Could you check a few things on this model? Use its own coordinates, in mm. Round coordinates to 2 decimals unless told otherwise and drop trailing zeros. Loops run counter-clockwise (first coordinate to the right, second up) from the corner with the lowest first, then second, coordinate; pieces in that order, holes last. Notation, with made-up numbers: (84.5, 17) - (138.5, 17) arc R21 ccw to (138.5, 40) - close; hole circle Ø10 at (0.5, 22.25). An arc over 180 degrees is marked (long way). Answer as CSV lines item,"result". Start each with the question number.
1) Suppose I cut it at B-B, the plane x = 45. Write out the boundary of the cut face in (y, z), then the cut area to 3 significant figures.
2) Suppose I cut it at D-D, the plane x = -10. Write out the boundary of the cut face in (y, z).
3) Please list where these lines run through material, in increasing order: line 1 along Z through (x, y) = (-38, 3.1); line 2 along Z through (x, y) = (-29, 1.2); line 3 along X through (y, z) = (1.35, 27).
4) Suppose I cut it at A-A, the plane z = -10. Write out the boundary of the cut face in (x, y).
5) I'm going to push flat-ended pins straight in: pin 1 Ø1 at (x, y) = (42, 3.5) entering from -Z; pin 2 Ø1.4 at (x, y) = (0, 2.5) entering from +Z. Where does each tip first touch, or does it pass through?
6) Suppose I cut it at C-C, the plane y = 2.95. Count the separate pieces of the cut face and the enclosed holes in it, then the cut area to 3 significant figures.
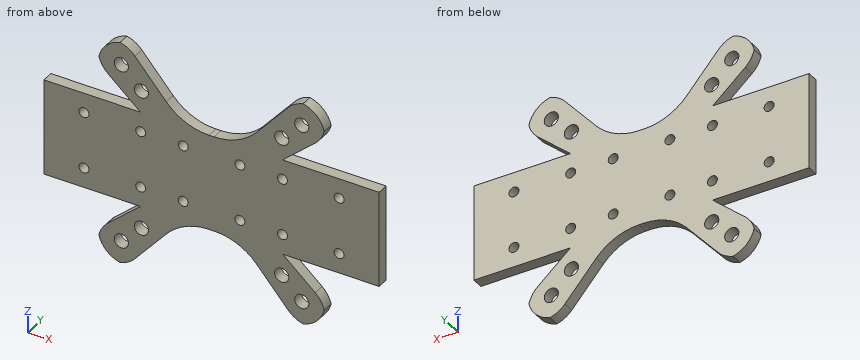
```python
from build123d import *

# Parameters (mm, degrees)
SKETCH1_W           = 80
SKETCH1_H           = 80
SKETCH1_R           = 2.5
SKETCH1_R_2         = 1.75
BOSS_EXTRUDE1_DEPTH = 4
CUT_EXTRUDE2_DEPTH  = 57.709787515
FILLET1_R           = 10
FILLET2_R           = 20
BOSS_EXTRUDE3_DEPTH = 4
SKETCH6_R           = 1.75
CUT_EXTRUDE3_DEPTH  = 4


with BuildPart() as part:
    # Sketch1 → Boss-Extrude1 (new body)
    with BuildSketch(Plane(origin=(0, 0, 0), x_dir=(1, 0, 0), z_dir=(0, 1, 0))):
        Rectangle(SKETCH1_W, SKETCH1_H)
        with Locations(Location((-24.748737342, 24.748737342, 0), (0, 0, 270))):
            Circle(SKETCH1_R, mode=Mode.SUBTRACT)
        with Locations(Location((24.748737342, 24.748737342, 0), (0, 0, 270))):
            Circle(SKETCH1_R, mode=Mode.SUBTRACT)
        with Locations(Location((24.748737342, -24.748737342, 0), (0, 0, 270))):
            Circle(SKETCH1_R, mode=Mode.SUBTRACT)
        with Locations(Location((-24.748737342, -24.748737342, 0), (0, 0, 270))):
            Circle(SKETCH1_R, mode=Mode.SUBTRACT)
        with Locations(Location((-10, 10, 0), (0, 0, 270))):
            Circle(SKETCH1_R_2, mode=Mode.SUBTRACT)
        with Locations(Location((10, 10, 0), (0, 0, 270))):
            Circle(SKETCH1_R_2, mode=Mode.SUBTRACT)
        with Locations(Location((10, -10, 0), (0, 0, 270))):
            Circle(SKETCH1_R_2, mode=Mode.SUBTRACT)
        with Locations(Location((-10, -10, 0), (0, 0, 270))):
            Circle(SKETCH1_R_2, mode=Mode.SUBTRACT)
        with Locations(Location((31.819805153, 31.819805153, 0), (0, 0, 270))):
            Circle(SKETCH1_R, mode=Mode.SUBTRACT)
        with Locations(Location((-31.819805153, 31.819805153, 0), (0, 0, 270))):
            Circle(SKETCH1_R, mode=Mode.SUBTRACT)
        with Locations(Location((-31.819805153, -31.819805153, 0), (0, 0, 270))):
            Circle(SKETCH1_R, mode=Mode.SUBTRACT)
        with Locations(Location((31.819805153, -31.819805153, 0), (0, 0, 270))):
            Circle(SKETCH1_R, mode=Mode.SUBTRACT)
    extrude(amount=BOSS_EXTRUDE1_DEPTH)

    # Sketch2 → Cut-Extrude2 (cut, through all)
    with BuildSketch(Plane(origin=(0, 4, 0), x_dir=(1, 0, 0), z_dir=(0, 1, 0))):
        Polygon((-40, 30), (-40, -30), (-17, -10), (-17, 10), align=None)
        Polygon((30, 40), (-30, 40), (-10, 17), (10, 17), align=None)
        Polygon((40, -30), (40, 30), (17, 10), (17, -10), align=None)
        Polygon((-30, -40), (30, -40), (10, -17), (-10, -17), align=None)
    extrude(amount=-CUT_EXTRUDE2_DEPTH, mode=Mode.SUBTRACT)

    # Fillet1
    # the kernel refuses this fillet: 10 mm, written as the material it takes off along each edge
    with BuildSketch(Plane(origin=(-30, 15.390762292, 40), x_dir=(-1, 0, 0), z_dir=(0, -1, 0)), Plane(origin=(-40, 15.390762292, 30), x_dir=(0.754605522163505, 0, -0.6561787149247863), z_dir=(0, -1, 0)), Plane(origin=(-40, 15.390762292, -30), x_dir=(0, 0, -1), z_dir=(0, -1, 0)), Plane(origin=(-30, 15.390762292, -40), x_dir=(0.6561787149247871, 0, 0.7546055221635043), z_dir=(0, -1, 0)), Plane(origin=(30, 15.390762292, -40), x_dir=(1, 0, 0), z_dir=(0, -1, 0)), Plane(origin=(40, 15.390762292, -30), x_dir=(-0.7546055221635045, 0, 0.6561787149247867), z_dir=(0, -1, 0)), Plane(origin=(40, 15.390762292, 30), x_dir=(0, 0, 1), z_dir=(0, -1, 0))) as fillet1_piece_1:
        with BuildLine():
            CenterArc((FILLET1_R * 0.455630491663, FILLET1_R), FILLET1_R, 221.009086902, 48.990913098)
            Line((-FILLET1_R * 0.2989750305, FILLET1_R * 0.343821285075), (0, 0))
            Line((0, 0), (FILLET1_R * 0.455630491663, 0))
        make_face()
    extrude(amount=26.781524583, mode=Mode.SUBTRACT)
    with BuildSketch(Plane(origin=(-40, -25, 40), x_dir=(0, 0, -1), z_dir=(0, 1, 0)), Plane(origin=(-40, -25, -40), x_dir=(1, 0, 0), z_dir=(0, 1, 0)), Plane(origin=(40, -25, -40), x_dir=(0, 0, 1), z_dir=(0, 1, 0)), Plane(origin=(40, -25, 40), x_dir=(-1, 0, 0), z_dir=(0, 1, 0))) as fillet1_piece_2:
        with BuildLine():
            CenterArc((FILLET1_R, -FILLET1_R), FILLET1_R, 90, 90)
            Line((0, -FILLET1_R), (0, 0))
            Line((0, 0), (FILLET1_R, 0))
        make_face()
    extrude(amount=54, mode=Mode.SUBTRACT)
    with BuildSketch(Plane(origin=(30, 15.390762292, 40), x_dir=(1, 0, 0), z_dir=(0, -1, 0))) as fillet1_piece_3:
        with BuildLine():
            CenterArc((FILLET1_R * 0.455630491663, -FILLET1_R), FILLET1_R, 90, 48.990913098)
            Line((-FILLET1_R * 0.2989750305, -FILLET1_R * 0.343821285075), (0, 0))
            Line((0, 0), (FILLET1_R * 0.455630491663, 0))
        make_face()
    extrude(amount=26.781524583, mode=Mode.SUBTRACT)

    # Fillet2
    fillet2_edges = [part.edges().sort_by_distance(p)[0] for p in [
        (10, 2, 17),
        (-10, 2, 17),
        (-17, 2, 10),
        (-17, 2, -10),
        (17, 2, -10),
        (17, 2, 10),
        (-10, 2, -17),
        (10, 2, -17),
    ]]
    fillet(fillet2_edges, radius=FILLET2_R)

    # Sketch5 → Boss-Extrude3 (add)
    with BuildSketch(Plane(origin=(0, 4, 0), x_dir=(1, 0, 0), z_dir=(0, 1, 0))):
        Polygon((-0.887390167, 17), (13.289046487, 12.123524967), (13.289046487, -13.496190448), (-0.887390167, -17), (59.112609833, -17), (59.112609833, 17), align=None)
    boss_extrude3 = extrude(amount=-BOSS_EXTRUDE3_DEPTH)

    # Sketch6 → Cut-Extrude3 (cut)
    with BuildSketch(Plane(origin=(0, 4, 0), x_dir=(1, 0, 0), z_dir=(0, 1, 0))):
        with Locations(Location((25, 10, 0), (0, 0, 270))):
            Circle(SKETCH6_R)
        with Locations(Location((45, 10, 0), (0, 0, 270))):
            Circle(SKETCH6_R)
        with Locations(Location((25, -10, 0), (0, 0, 270))):
            Circle(SKETCH6_R)
        with Locations(Location((45, -10, 0), (0, 0, 270))):
            Circle(SKETCH6_R)
    cut_extrude3 = extrude(amount=-CUT_EXTRUDE3_DEPTH, mode=Mode.SUBTRACT)

    # Mirror1: Boss-Extrude3, Cut-Extrude3 across plane
    add(boss_extrude3.mirror(Plane(origin=(0, 0, 0), x_dir=(0, 0, 1), z_dir=(1, 0, 0))))
    add(cut_extrude3.mirror(Plane(origin=(0, 0, 0), x_dir=(0, 0, 1), z_dir=(1, 0, 0))), mode=Mode.SUBTRACT)


solid = part.part
```
Filled sheet:
1,outline,"(0, -17) - (4, -17) - (4, -11.75) - (0, -11.75) - close; (0, -8.25) - (4, -8.25) - (4, 8.25) - (0, 8.25) - close; (0, 11.75) - (4, 11.75) - (4, 17) - (0, 17) - close"
1,area,"108 mm²"
2,outline,"(0, -19.2) - (4, -19.2) - (4, -11.75) - (0, -11.75) - close; (0, -8.25) - (4, -8.25) - (4, 8.25) - (0, 8.25) - close; (0, 11.75) - (4, 11.75) - (4, 19.2) - (0, 19.2) - close"
3,line 1,"-36 to -28.56, -17 to 17, 28.56 to 36"
3,line 2,"-38.31 to -20.43, -17 to 17, 20.43 to 38.31"
3,line 3,"-36.55 to -25.84, -23.66 to -18.7, 18.7 to 23.66, 25.84 to 36.55"
4,outline,"(-59.11, 0) - (-46.75, 0) - (-46.75, 4) - (-59.11, 4) - close; (-43.25, 0) - (-26.75, 0) - (-26.75, 4) - (-43.25, 4) - close; (-23.25, 0) - (-11.75, 0) - (-11.75, 4) - (-23.25, 4) - close; (-8.25, 0) - (8.25, 0) - (8.25, 4) - (-8.25, 4) - close; (11.75, 0) - (23.25, 0) - (23.25, 4) - (11.75, 4) - close; (26.75, 0) - (43.25, 0) - (43.25, 4) - (26.75, 4) - close; (46.75, 0) - (59.11, 0) - (59.11, 4) - (46.75, 4) - close"
5,pin 1,"z = -17"
5,pin 2,"z = 17"
6,separate pieces,"1"
6,enclosed holes,"20"
6,area,"5,140 mm²"
